Geometry check sheet. Reference: the model listing, model coordinates, mm. A direction names the side the tool comes from. Round coordinates to 2 decimals unless told otherwise and drop trailing zeros. Write each loop counter-clockwise with the first axis right and the second up, starting at its lowest first coordinate (ties: lowest second). Pieces come first, ordered by that corner, then holes. Notation, with made-up numbers: (68.25, 76) -> (113.25, 76) arc R21 ccw to (113.25, 111) -> close; hole circle Ø11 at (78, 4.5). An arc over 180 degrees is marked (long way). Return JSON: item names as keys, results as strings. Group by question number.
from build123d import *

# Parameters (mm, degrees)
SKETCH1_R           = 19.05
BOSS_EXTRUDE1_DEPTH = 17.78
SKETCH2_R           = 10.16
CUT_EXTRUDE1_DEPTH  = 1.27
FILLET1_R           = 2.54
FILLET2_R           = 2.54
SKETCH3_R           = 20.32
BOSS_EXTRUDE2_DEPTH = 12.7
FILLET3_R           = 2.54
SKETCH4_R           = 17.78
BOSS_EXTRUDE3_DEPTH = 2.54
SKETCH5_R           = 13.97
BOSS_EXTRUDE4_DEPTH = 1.6764
FILLET5_R           = 0.635
SKETCH6_R           = 11.43
CUT_EXTRUDE2_DEPTH  = 33.02
BOSS_EXTRUDE6_DEPTH = 10.414
SKETCH9_W           = 5.530491266
SKETCH9_H           = 40.61393848
BOSS_EXTRUDE7_DEPTH = 33.02
FILLET6_START       = -20.30755603
FILLET6_DEPTH       = 40.61393848
FILLET6_START_2     = 30.48
FILLET6_2_DEPTH     = 2.52


with BuildPart() as part:
    # Sketch1 → Boss-Extrude1 (new body)
    with BuildSketch(Plane.XY):
        Circle(SKETCH1_R)
    extrude(amount=BOSS_EXTRUDE1_DEPTH)

    # Sketch2 → Cut-Extrude1 (cut)
    with BuildSketch(Plane(origin=(0, 0, 0), x_dir=(-1, 0, 0), z_dir=(0, 0, -1))):
        Circle(SKETCH2_R)
    extrude(amount=-CUT_EXTRUDE1_DEPTH, mode=Mode.SUBTRACT)

    # Fillet1
    # the kernel refuses this fillet: 2.54 mm, written as the material it takes off along each edge
    with BuildSketch(Plane(origin=(0, 0, 0), x_dir=(-1, 0, 0), z_dir=(0, -1, 0))) as fillet1_piece_1:
        with BuildLine():
            CenterArc((12.359704526, -2.54), FILLET1_R, 90, 60)
            Line((10.16, -1.27), (10.116005909, -1.2446))
            ThreePointArc((10.116005909, -1.2446), (10.1092, -0.635), (10.1092, 0))
            Line((10.1092, 0), (10.16, 0.0508))
            Line((10.16, 0.0508), (12.359704526, 0.0508))
            Line((12.359704526, 0.0508), (12.359704526, 0))
        make_face()
    revolve(axis=Axis((0, 0, 0), (0, 0, -1)), mode=Mode.SUBTRACT)

    # Fillet2
    fillet2_edges = [part.edges().sort_by_distance(p)[0] for p in [
        (-19.05, 0, 0),
    ]]
    fillet(fillet2_edges, radius=FILLET2_R)

    # Sketch3 → Boss-Extrude2 (add)
    with BuildSketch(Plane.XY.offset(17.78)):
        Circle(SKETCH3_R)
    extrude(amount=BOSS_EXTRUDE2_DEPTH)

    # Fillet3
    # the kernel refuses this fillet: 2.54 mm, written as the material it takes off along each edge
    with BuildSketch(Plane(origin=(0, 0, 17.78), x_dir=(1, 0, 0), z_dir=(0, -1, 0))) as fillet3_piece_1:
        with BuildLine():
            CenterArc((17.78, 2.199704526), FILLET3_R, 300, 60)
            Line((19.05, 0), (19.0754, -0.043994091))
            ThreePointArc((19.0754, -0.043994091), (19.685, -0.0508), (20.32, -0.0508))
            Line((20.32, -0.0508), (20.3708, 0))
            Line((20.3708, 0), (20.3708, 2.199704526))
            Line((20.3708, 2.199704526), (20.32, 2.199704526))
        make_face()
    revolve(axis=Axis((0, 0, 17.78), (0, 0, 1)), mode=Mode.SUBTRACT)

    # Sketch4 → Boss-Extrude3 (add)
    with BuildSketch(Plane.XY.offset(30.48)):
        Circle(SKETCH4_R)
    extrude(amount=BOSS_EXTRUDE3_DEPTH)

    # Sketch5 → Boss-Extrude4 (add)
    with BuildSketch(Plane.XY.offset(33.02)):
        Circle(SKETCH5_R)
    extrude(amount=BOSS_EXTRUDE4_DEPTH)

    # Fillet5
    fillet5_edges = [part.edges().sort_by_distance(p)[0] for p in [
        (-17.78, 0, 33.02),
        (-13.97, 0, 34.6964),
    ]]
    fillet(fillet5_edges, radius=FILLET5_R)

    # Sketch6 → Cut-Extrude2 (cut)
    with BuildSketch(Plane.XY.offset(34.6964)):
        Circle(SKETCH6_R)
    extrude(amount=-CUT_EXTRUDE2_DEPTH, mode=Mode.SUBTRACT)

    # Sketch7 → Boss-Extrude6 (add)
    with BuildSketch(Plane.XY.offset(30.48)):
        with BuildLine():
            Line((0.71103311, -20.30755603), (26.11103311, -20.30755603))
            Line((26.11103311, -20.30755603), (26.11103311, 20.30638245))
            Line((26.11103311, 20.30638245), (0.743795542, 20.30638245))
            Line((0.743795542, 20.30638245), (0.743795542, 19.03638245))
            add(Edge.make_bspline(
                [(0.71103311, -19.03755603), (10.719056995, -19.88065927), (29.921844126, -0.322882605), (10.700257888, 19.398993092), (0.743795542, 19.03638245)],
                knots=[0, 0, 0, 0, 0.495916673, 1, 1, 1, 1], degree=3))
            Line((0.71103311, -19.03755603), (0.71103311, -20.30755603))
        make_face()
    extrude(amount=-BOSS_EXTRUDE6_DEPTH)

    # Sketch9 → Boss-Extrude7 (add)
    with BuildSketch(Plane.XY.offset(30.48)):
        with Locations((23.345787477, -0.00058679)):
            Rectangle(SKETCH9_W, SKETCH9_H)
    extrude(amount=BOSS_EXTRUDE7_DEPTH)

    # Fillet6: read off the stored shape, not the designer's step
    # Fillet6 outline → Fillet6 (add)
    with BuildSketch(Plane(origin=(0, 0, 0), x_dir=(1, 0, 0), z_dir=(0, 1, 0)).offset(FILLET6_START)):
        with BuildLine():
            Line((20.580541844, -30.48), (18.040541844, -30.48))
            ThreePointArc((18.040541844, -30.48), (19.836593068, -31.223948776), (20.580541844, -33.02))
            Line((20.580541844, -33.02), (20.580541844, -30.48))
        make_face()
    extrude(amount=FILLET6_DEPTH)

    # Fillet6 2 outline → Fillet6 2 (cut)
    with BuildSketch(Plane.XY.offset(FILLET6_START_2)):
        with BuildLine():
            add(Edge.make_bspline(
                [(20.315186876, -0.442246776), (20.310692243, -1.040693916), (20.270518605, -1.638988681), (20.196745769, -2.234694689)],
                knots=[0.504083327, 0.504083327, 0.504083327, 0.504083327, 0.534555468, 0.534555468, 0.534555468, 0.534555468], degree=3))
            ThreePointArc((20.315186876, -0.442246776), (20.275783315, -1.339780197), (20.196745769, -2.234694689))
        make_face()
    extrude(amount=FILLET6_2_DEPTH, mode=Mode.SUBTRACT)


solid = part.part
1) Sectioned sample at D-D on x = 22. Enter the section's corners in (y, z), and give its area (3 significant figures).
2) Go/stop test with flat-tipped pins: P1, Ø18.5, axis at x = 0, y = 0, coming from the -Z side; P2, Ø11.5, axis at x = -1, y = 0.5, coming from the +Z side; P3, Ø10, axis at x = -12, y = 12, coming from the +Z side. Record where each tip stops, or that it passes through.
3) Tool access check on faces 4 (the face through (-1.82, 13.85, 33.53)), 5 (the face through (10, 6, 34.696)), 6 (the face through (0, 0, 1.27)). Record the directions out of +Z, -Z, +X, -X, +Y, -Y that give a thin tool (end or side, any length) a straight path to the whole face; none if there is none.
4) Material ranges on probe 1 along Y at (x, z) = (0, 8); probe 2 along Y at (x, z) = (0, 25); probe 3 along Z at (x, y) = (12, 4), recorded low to high. Write a range as [from, to].
5) Sectioned sample at C-C on z = 25. State how many separate pieces and enclosed holes the cut face has, and give its area (3 significant figures).
6) Sectioned sample at B-B on z = 13. Enter the section's corners in (x, y), and give its area (3 significant figures).
7) Mould release check, pull along X, two halves, no side actions. Record for faces 1 (the face through (23, 0, 63.5)), 2 (the face through (10.902, 3.433, 18.418)), 3 (the face through (-15.12, -11.59, 10.05)): +X half, -X half, draft (parallel to the pull), parting line (faces both ways), or undercut.
Evaluation:
{
 "1": {"outline": "(-20.31, 20.07) -> (20.31, 20.07) -> (20.31, 63.5) -> (-20.31, 63.5) -> close", "area": "1,760 mm2"},
 "2": {"P1": "stops at z = 1.27", "P2": "stops at z = 1.68", "P3": "stops at z = 34.7"},
 "3": {"face 4": "+Z", "face 5": "+Z, -X, +Y, -Y", "face 6": "-Z"},
 "4": {"probe 1": "y = [-19.05, -11.43], [11.43, 19.05]", "probe 2": "y = [-20.32, -11.43], [11.43, 20.32]", "probe 3": "z = [0, 34.7]"},
 "5": {"separate pieces": "1", "enclosed holes": "2", "area": "1,300 mm2"},
 "6": {"outline": "circle Ø38.1 at (0, 0); hole circle Ø22.86 at (0, 0)", "area": "730 mm2"},
 "7": {"face 1": "draft", "face 2": "undercut", "face 3": "parting line"}
}
